```python
from build123d import *

# Parameters (mm, degrees)
SKETCH1_W           = 304.8
SKETCH1_H           = 152.4
BOSS_EXTRUDE1_DEPTH = 5.334
SKETCH2_R           = 3.175
CUT_EXTRUDE1_DEPTH  = 10
SKETCH4_R           = 2.676950891
SKETCH4_R_2         = 2.665674254
SKETCH4_R_3         = 2.530032229
SKETCH4_R_4         = 2.5353316
CUT_EXTRUDE3_DEPTH  = 252.586384458
SKETCH5_W           = 5.334
SKETCH5_H           = 6.35
SKETCH5_H_2         = 5.207
CUT_EXTRUDE4_DEPTH  = 252.586384458
SKETCH8_W           = 76.2
SKETCH8_H           = 34.29
CUT_EXTRUDE5_DEPTH  = 252.586384458
SKETCH10_W          = 76.2
SKETCH10_H          = 1.778250289
SKETCH10_H_2        = 2.019413315
CUT_EXTRUDE7_DEPTH  = 252.586384458
SKETCH11_W          = 76.121070341
SKETCH11_H          = 36.949838164
CUT_EXTRUDE8_DEPTH  = 252.586384458
SKETCH12_W          = 14.224
SKETCH12_H          = 12.638991695
CUT_EXTRUDE9_DEPTH  = 252.586384458
SKETCH13_W          = 18.627313318
SKETCH13_H          = 34.653875248
CUT_EXTRUDE10_DEPTH = 252.586384458
CUT_EXTRUDE11_DEPTH = 252.586384458


with BuildPart() as part:
    # Sketch1 → Boss-Extrude1 (new body)
    with BuildSketch(Plane(origin=(0, 0, 0), x_dir=(1, 0, 0), z_dir=(0, 1, 0))):
        with Locations((-63.754910023, -52.424694992)):
            Rectangle(SKETCH1_W, SKETCH1_H)
    extrude(amount=BOSS_EXTRUDE1_DEPTH)

    # Sketch2 → Cut-Extrude1 (cut)
    with BuildSketch(Plane(origin=(0, 5.334, 0), x_dir=(1, 0, 0), z_dir=(0, 1, 0))):
        with Locations(Location((-201.154910023, -113.624694992, 0), (0, 0, 270))):
            Circle(SKETCH2_R)
        with Locations(Location((-201.154910023, 8.775305008, 0), (0, 0, 270))):
            Circle(SKETCH2_R)
        with Locations(Location((73.468003191, -112.082866523, 0), (0, 0, 270))):
            Circle(SKETCH2_R)
        with Locations(Location((72.093654241, 10.309417404, 0), (0, 0, 270))):
            Circle(SKETCH2_R)
    extrude(amount=-CUT_EXTRUDE1_DEPTH, mode=Mode.SUBTRACT)

    # Sketch4 → Cut-Extrude3 (cut, through all)
    with BuildSketch(Plane(origin=(0, 5.334, 0), x_dir=(1, 0, 0), z_dir=(0, 1, 0))):
        with Locations(Location((-91.687860004, -24.357805151, 0), (0, 0, 270))):
            Circle(SKETCH4_R)
        with Locations(Location((-35.688020182, -24.491745011, 0), (0, 0, 270))):
            Circle(SKETCH4_R_2)
        with Locations(Location((-43.855422124, -94.472410523, 0), (0, 0, 270))):
            Circle(SKETCH4_R_3)
        with Locations(Location((-83.855307711, -94.376739195, 0), (0, 0, 270))):
            Circle(SKETCH4_R_4)
    extrude(amount=-CUT_EXTRUDE3_DEPTH, mode=Mode.SUBTRACT)

    # Sketch5 → Cut-Extrude4 (cut, through all)
    with BuildSketch(Plane(origin=(0, 5.334, 0), x_dir=(1, 0, 0), z_dir=(0, 1, 0))):
        with Locations((-204.597910023, -77.824694992)):
            Rectangle(SKETCH5_W, SKETCH5_H)
        with Locations((-204.597910023, -27.024694992)):
            Rectangle(SKETCH5_W, SKETCH5_H)
        with Locations((-175.133910023, -26.453194992)):
            Rectangle(SKETCH5_W, SKETCH5_H_2)
        with Locations((-175.133910023, -78.396194992)):
            Rectangle(SKETCH5_W, SKETCH5_H_2)
        with Locations((77.088089977, -77.824694992)):
            Rectangle(SKETCH5_W, SKETCH5_H)
        with Locations((47.624089977, -78.396194992)):
            Rectangle(SKETCH5_W, SKETCH5_H_2)
        with Locations((77.088089977, -27.024694992)):
            Rectangle(SKETCH5_W, SKETCH5_H)
        with Locations((47.624089977, -26.453194992)):
            Rectangle(SKETCH5_W, SKETCH5_H_2)
    extrude(amount=-CUT_EXTRUDE4_DEPTH, mode=Mode.SUBTRACT)

    # Sketch8 → Cut-Extrude5 (cut, through all)
    with BuildSketch(Plane(origin=(0, 5.334, 0), x_dir=(1, 0, 0), z_dir=(0, 1, 0))):
        with Locations((36.321089977, -52.424694992)):
            Rectangle(SKETCH8_W, SKETCH8_H)
    extrude(amount=-CUT_EXTRUDE5_DEPTH, mode=Mode.SUBTRACT)

    # Sketch10 → Cut-Extrude7 (cut, through all)
    with BuildSketch(Plane(origin=(0, 5.334, 0), x_dir=(1, 0, 0), z_dir=(0, 1, 0))):
        with Locations((36.321089977, -70.458820137)):
            Rectangle(SKETCH10_W, SKETCH10_H)
        with Locations((36.321089977, -34.269988334)):
            Rectangle(SKETCH10_W, SKETCH10_H_2)
    extrude(amount=-CUT_EXTRUDE7_DEPTH, mode=Mode.SUBTRACT)

    # Sketch11 → Cut-Extrude8 (cut, through all)
    with BuildSketch(Plane(origin=(0, 5.334, 0), x_dir=(1, 0, 0), z_dir=(0, 1, 0))):
        with Locations((-163.870374853, -52.409398233)):
            Rectangle(SKETCH11_W, SKETCH11_H)
    extrude(amount=-CUT_EXTRUDE8_DEPTH, mode=Mode.SUBTRACT)

    # Sketch12 → Cut-Extrude9 (cut, through all)
    with BuildSketch(Plane(origin=(0, 5.334, 0), x_dir=(1, 0, 0), z_dir=(0, 1, 0))):
        with Locations((-209.042910023, -52.397947161)):
            Rectangle(SKETCH12_W, SKETCH12_H)
    extrude(amount=-CUT_EXTRUDE9_DEPTH, mode=Mode.SUBTRACT)

    # Sketch13 → Cut-Extrude10 (cut, through all)
    with BuildSketch(Plane(origin=(0, 5.334, 0), x_dir=(1, 0, 0), z_dir=(0, 1, 0))):
        with Locations((-92.547768292, -53.386052829)):
            Rectangle(SKETCH13_W, SKETCH13_H)
    extrude(amount=-CUT_EXTRUDE10_DEPTH, mode=Mode.SUBTRACT)

    # Sketch14 → Cut-Extrude11 (cut, through all)
    with BuildSketch(Plane(origin=(0, 5.334, 0), x_dir=(1, 0, 0), z_dir=(0, 1, 0))):
        Polygon((74.421089977, -52.304113479), (74.421089977, -58.539435279), (88.645089977, -58.539435279), (88.645089977, -45.874866735), (74.421089977, -45.874866735), align=None)
    extrude(amount=-CUT_EXTRUDE11_DEPTH, mode=Mode.SUBTRACT)


solid = part.part
```
Could you check a few things on this model? Use its own coordinates, in mm. Coordinates: 2 decimals unless noted, no trailing zeros. Loops run counter-clockwise (first coordinate to the right, second up) from the corner with the lowest first, then second, coordinate; pieces in that order, holes last. Notation, with made-up numbers: M 10.5,29 L 33.5,29 A19 cw 33.5,49 Z; hole C 22,-36.75 d7. An arc over 180 degrees is marked long. Put each result on its own line as item: value. Start each with the question number.
(1) Suppose I cut it at B-B on x = 11. Please give me the cut outline in (y, z), then the cut area to 3 significant figures.
(2) I need wall thicknesses on line 1 (Z direction, x = -201.5, y = 1.45); line 2 (X direction, y = 4.25, z = 37); line 3 (Z direction, x = 4, y = 4.2). Which ranges of each line are inside material? Lowest first, please. Write a range as from..to.
(3) Suppose I cut it at C-C on y = 4.35. Count the separate pieces of the cut face and the enclosed holes in it, then the cut area to 3 significant figures.
(4) Thinking about a two-plate mould opening in X: for faces 1 (the face through (-125.81, 3, 53)), 2 (the face through (-66, 5.334, 51)), which applies, pulls with the +X half, pulls with the -X half, needs draft (parallel to the pull), parting line crosses it, or undercut?
(5) Will this pin go through, and if not, where does the flat tip stop? P1, Ø3, axis at x = -43.86, z = 94.47, coming from the +Y side.
(6) Suppose I cut it at A-A on x = -131.5. Please give me the cut outline in (y, z).
Solutions:
1. outline: M 0,-23.78 L 5.33,-23.78 L 5.33,33.26 L 0,33.26 Z; M 0,71.35 L 5.33,71.35 L 5.33,128.62 L 0,128.62 Z
1. area: 610 mm2
2. line 1: z = -23.78..-11.93, -5.62..33.93, 70.88..110.47, 116.78..128.62
2. line 2: x = -216.15..-201.93, -125.81..-101.86, -83.23..-1.78, 74.42..88.65
2. line 3: z = -23.78..33.26, 71.35..128.62
3. separate pieces: 1
3. enclosed holes: 17
3. area: 39,300 mm2
4. face 1: undercut
4. face 2: needs draft
5. P1: passes through
6. outline: M 0,-23.78 L 5.33,-23.78 L 5.33,33.93 L 0,33.93 Z; M 0,70.88 L 5.33,70.88 L 5.33,128.62 L 0,128.62 Z
